from build123d import *

# Parameters (mm, degrees)
SKETCH1_W           = 90
SKETCH1_H           = 160
BOSS_EXTRUDE1_DEPTH = 5
SKETCH2_W           = 90
SKETCH2_H           = 160
SKETCH2_W_2         = 85
SKETCH2_H_2         = 155
BOSS_EXTRUDE2_DEPTH = 10
SKETCH3_W           = 85
SKETCH3_H           = 8.25
SKETCH3_R           = 1.5
BOSS_EXTRUDE3_DEPTH = 7
SKETCH4_W           = 45
SKETCH4_H           = 39.175
SKETCH4_H_2         = 10
SKETCH4_R           = 2.5
BOSS_EXTRUDE4_DEPTH = 7
FILLET1_R           = 3
SKETCH5_R           = 2.5
SKETCH5_R_2         = 2.55926668
SKETCH5_R_3         = 1.5
CUT_EXTRUDE1_DEPTH  = 119.276665608


with BuildPart() as part:
    # Sketch1 → Boss-Extrude1 (new body)
    with BuildSketch(Plane(origin=(0, 0, 0), x_dir=(1, 0, 0), z_dir=(0, 1, 0))):
        with Locations((1.726862302, -28.194130926)):
            Rectangle(SKETCH1_W, SKETCH1_H)
    extrude(amount=BOSS_EXTRUDE1_DEPTH)

    # Sketch2 → Boss-Extrude2 (add)
    with BuildSketch(Plane(origin=(0, 5, 0), x_dir=(1, 0, 0), z_dir=(0, 1, 0))):
        with Locations((1.726862302, -28.194130926)):
            Rectangle(SKETCH2_W, SKETCH2_H)
        with Locations((1.726862302, -28.194130926)):
            Rectangle(SKETCH2_W_2, SKETCH2_H_2, mode=Mode.SUBTRACT)
    extrude(amount=BOSS_EXTRUDE2_DEPTH)

    # Sketch3 → Boss-Extrude3 (add)
    with BuildSketch(Plane(origin=(0, 5, 0), x_dir=(1, 0, 0), z_dir=(0, 1, 0))):
        with Locations((1.726862302, -101.569130926)):
            Rectangle(SKETCH3_W, SKETCH3_H)
        with Locations(Location((-36.023137698, -100.944130926, 0), (0, 0, 270))):
            Circle(SKETCH3_R, mode=Mode.SUBTRACT)
        with Locations(Location((39.476862302, -100.944130926, 0), (0, 0, 270))):
            Circle(SKETCH3_R, mode=Mode.SUBTRACT)
    extrude(amount=BOSS_EXTRUDE3_DEPTH)

    # Sketch4 → Boss-Extrude4 (add)
    # profile 1 of 2: a face of its own
    with BuildSketch(Plane(origin=(0, 5, 0), x_dir=(1, 0, 0), z_dir=(0, 1, 0))):
        with Locations((-18.273137698, 29.718369074)):
            Rectangle(SKETCH4_W, SKETCH4_H)
    # profile 2 of 2: a face of its own
    with BuildSketch(Plane(origin=(0, 5, 0), x_dir=(1, 0, 0), z_dir=(0, 1, 0))):
        with Locations((-18.273137698, 5.130869074)):
            Rectangle(SKETCH4_W, SKETCH4_H_2)
        with Locations(Location((-29.023137698, 5.130869074, 0), (0, 0, 90))):
            Circle(SKETCH4_R, mode=Mode.SUBTRACT)
        with Locations(Location((-19.023137698, 5.130869074, 0), (0, 0, 90))):
            Circle(SKETCH4_R, mode=Mode.SUBTRACT)
    extrude(amount=BOSS_EXTRUDE4_DEPTH)

    # Fillet1
    fillet1_edges = [part.edges().sort_by_distance(p)[0] for p in [
        (-43.273137698, 7.5, -51.805869074),
        (46.726862302, 7.5, -51.805869074),
        (46.726862302, 7.5, 108.194130926),
        (-43.273137698, 7.5, 108.194130926),
    ]]
    fillet(fillet1_edges, radius=FILLET1_R)

    # Sketch5 → Cut-Extrude1 (cut, through all)
    with BuildSketch(Plane(origin=(0, 5, 0), x_dir=(1, 0, 0), z_dir=(0, 1, 0))):
        with Locations(Location((-19.023137698, 5.130869074, 0), (0, 0, 90))):
            Circle(SKETCH5_R)
        with Locations(Location((-29.023137698, 5.130869074, 0), (0, 0, 270))):
            Circle(SKETCH5_R_2)
        with Locations(Location((-36.023137698, -100.944130926, 0), (0, 0, 270))):
            Circle(SKETCH5_R_3)
        with Locations(Location((39.476862302, -100.944130926, 0), (0, 0, 270))):
            Circle(SKETCH5_R_3)
    extrude(amount=-CUT_EXTRUDE1_DEPTH, mode=Mode.SUBTRACT)


solid = part.part
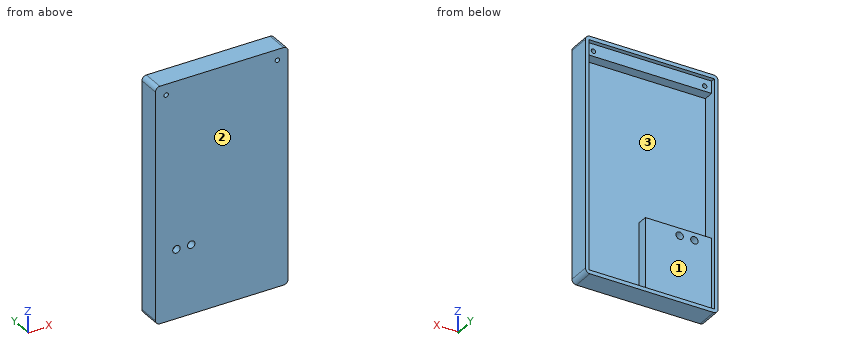
The model under review builds one solid part; all positions refer to its coordinate system, in mm. Face numbers are marked on the shaded views. Give positions to 0.01 mm unless a question says otherwise; leave off trailing zeros. Loops run counter-clockwise (first coordinate to the right, second up) from the corner with the lowest first, then second, coordinate; pieces in that order, holes last. Notation, with made-up numbers: (31.5, -14) -> (86.5, -14) arc R36 cw to (86.5, 23) -> close; hole circle Ø1 at (71, 6.25). An arc over 180 degrees is marked (long way). Answer as a JSON object with one key per item and string values. Group by question number.
Q1. Wall thickness on line 1 along X through (y, z) = (14, -42.5); line 2 along Z through (x, y) = (11, 10.5); line 3 along Z through (x, y) = (-26, 9.5): over which ranges is each line inside the solid? List them lowest first.
Q2. Draft analysis for pull direction X (two halves, no side actions). For the marked faces 1, 2 and 3, state which applies: pulls with the +X half, pulls with the -X half, needs draft (parallel to the pull), parting line crosses it, or undercut.
Q3. Insertion check: pin 1 (5 mm diameter, centred on x = -32, z = -6, fed in from +Y); pin 2 (10 mm diameter, centred on x = -19, z = 42, fed in from +Y). Each pin has a flat end and moves straight along its axis. Give the tip position at first contact, or say it passes through.
Q4. Take a section at C-C (z = 76). Write out the cut boundary in (x, y).
Q5. Take a section at A-A (y = 13.5). Write out the cut boundary in (x, z), plus the area to 3 significant figures.
Q6. Take a section at B-B (x = 25). Write out the cut boundary in (y, z).
Answer below:
{
 "1": {"line 1": "x = -43.27 to -40.77, 44.23 to 46.73", "line 2": "z = -51.81 to -49.31, 97.44 to 108.19", "line 3": "z = -51.81 to -0.13, 97.44 to 108.19"},
 "2": {"face 1": "undercut", "face 2": "needs draft", "face 3": "undercut"},
 "3": {"pin 1": "stops at y = 12", "pin 2": "stops at y = 5"},
 "4": {"outline": "(-43.27, 0) -> (46.73, 0) -> (46.73, 15) -> (44.23, 15) -> (44.23, 5) -> (-40.77, 5) -> (-40.77, 15) -> (-43.27, 15) -> close"},
 "5": {"outline": "(-43.27, -48.81) arc R3 ccw to (-40.27, -51.81) -> (43.73, -51.81) arc R3 ccw to (46.73, -48.81) -> (46.73, 105.19) arc R3 ccw to (43.73, 108.19) -> (-40.27, 108.19) arc R3 ccw to (-43.27, 105.19) -> close; hole (-40.77, -49.31) -> (44.23, -49.31) -> (44.23, 105.69) -> (-40.77, 105.69) -> close", "area": "1,220 mm2"},
 "6": {"outline": "(0, -51.81) -> (15, -51.81) -> (15, -49.31) -> (5, -49.31) -> (5, 97.44) -> (12, 97.44) -> (12, 105.69) -> (15, 105.69) -> (15, 108.19) -> (0, 108.19) -> close"}
}
